Autodesk Inventor part; units mm, degrees
ref_plane "YZ Plane" through (0, 0, 0) normal (1, 0, 0) x (0, 1, 0)
ref_plane "XZ Plane" through (0, 0, 0) normal (0, 1, 0) x (-1, 0, 0)
ref_plane "XY Plane" through (0, 0, 0) normal (0, 0, 1) x (1, 0, 0)
sketch "Sketch1" plane through (0, 0, 0) normal (0, 1, 0) x (-1, 0, 0)
  circle A0 centre (0, 0) radius 60 construction
  circle A1 centre (0, 0) radius 55 construction
  circle A2 centre (0, 55) radius 2.2
  arc A3 (5.2293, 59.7717) -> (-5.2293, 59.7717) centre (0, 0) ccw
  line L0 (0, 0) -> (5.2293, 59.7717) construction
  line L1 (0, 0) -> (60, 0) construction
  line L2 (0, 0) -> (-5.2293, 59.7717) construction
  line L3 (0, 24.4692) -> (0, -19) construction
  arc A4 (-4.7936, 54.7907) -> (4.7936, 54.7907) centre (0, 55) ccw
  line L4 (4.7936, 54.7907) -> (5.2293, 59.7717)
  line L5 (-5.2293, 59.7717) -> (-4.7936, 54.7907)
  circle A5 centre (0, 55) radius 3.9
  dimension "d0" = 120
  dimension "d1" = 110
  dimension "d2" = 4.4
  dimension "d4" = 10
  dimension "d5" = 5
  dimension "d8" = 7.8
extrude "Extrusion1" add sketch "Sketch1" along normal blind 25 contours L4 A4 L5 A3 | A5
extrude "Extrusion2" add sketch "Sketch1" along normal blind 26.9 and the other way blind 1.9 contours A5
fillet "Fillet1" radius 1.9 2 edges at (3.9, 26.9, 55) (3.9, -1.9, 55)
equation "\"d5\" = 0.5 * d4"
properties part number "Spacer"
For this review, take the finished solid that the model builds, in its own axes (mm). A direction names the side the tool comes from. Give positions to 0.01 mm unless a question says otherwise; leave off trailing zeros. Loops run counter-clockwise (first coordinate to the right, second up) from the corner with the lowest first, then second, coordinate; pieces in that order, holes last.
Item 1: Tool access review of faces 5 (the flat face through (-2.3, 0, 58.4)), 6 (the flat face through (5.014, 12.325, 57.316)): name each direction out of +Z, -Z, +X, -X, +Y, -Y from which nothing blocks a thin tool from reaching the whole face with its end or side.
Item 2: Insertion check: pin 1 (4 mm diameter, centred on y = 4.5, z = 55, fed in from +X); pin 2 (2 mm diameter, centred on x = -3, y = 15.5, fed in from -Z); pin 3 (5 mm diameter, centred on x = -3.5, y = 13.5, fed in from +Z). Each pin has a flat end and moves straight along its axis. Give the tip position at first contact, or say it passes through.
Item 3: Take a section at C-C, the plane x = 4.5. State the section outline as (y, z) points, and give its area (3 significant figures).
Item 4: Draft analysis for pull direction Z (two halves, no side actions). For faces 1 (the cylindrical face through (0, 12, 60)), 2 (the flat face through (-2.3, 25, 58.4)), 3 (the cylindrical face through (0.477, 12.702, 52.852)), 4 (the cylindrical face through (-0.103, 12.325, 50.203)), state which applies: +Z half, -Z half, draft (parallel to the pull), parting line (faces both ways), or undercut.
Item 5: For line 1 along Y through (x, z) = (-4.5, 58.25); line 2 along Z through (x, y) = (1.25, 13); line 3 along Y through (x, z) = (-3, 54.25), list the stretches that pass through material, from the lowest coordinate up.
Calculated:
1. face 5: -Y
1. face 6: -Z, +X, +Y, -Y
2. pin 1: stops at x = 4.99
2. pin 2: stops at z = 50.64
2. pin 3: stops at z = 59.99
3. outline: (0, 53.33) - (25, 53.33) - (25, 59.83) - (0, 59.83) - close
3. area: 162 mm2
4. face 1: +Z half
4. face 2: draft
4. face 3: undercut
4. face 4: -Z half
5. line 1: y = 0 to 25
5. line 2: z = 50.37 to 53.19, 56.81 to 59.99
5. line 3: y = -1.57 to 26.57
